Design review of the part shown in the three views and the two pictorial views. Dimensions are in mm from the part's minimum x, y and z. Round coordinates to 2 decimals unless told otherwise and drop trailing zeros. Write each loop counter-clockwise with the first axis right and the second up, starting at its lowest first coordinate (ties: lowest second). Pieces come first, ordered by that corner, then holes. Notation, with made-up numbers: (76, -4.75) -> (105, -4.75) arc R23 ccw to (105, 11.25) -> close; hole circle Ø11 at (52, 57). An arc over 180 degrees is marked (long way). Return JSON: item names as keys, results as strings. Group by question number.
1. Take a section at C-C, the plane x = 71.5. Write out the cut boundary in (y, z).
2. Take a section at B-B, the plane z = 27. Write out the cut boundary in (x, y).
3. Take a section at D-D, the plane y = 45.5. Write out the cut boundary in (x, z).
4. Take a section at A-A, the plane y = 27. Write out the cut boundary in (x, z).
5. Clearance check with flat-ended pins moving along their axes: P1, Ø5, axis at x = 98.5, z = 9.5, coming from the +Y side; P2, Ø3, axis at x = 69.5, y = 11, coming from the +Z side; P3, Ø4, axis at x = 71.5, y = 10, coming from the -Z side. State where each tip first meets the part, or that it passes through.
6. For line 1 along Z through (x, y) = (46, 27); line 2 along Y through (x, z) = (43, 17); line 3 along Z through (x, y) = (94.5, 33.5), list the stretches that pass through material, from the lowest coordinate up. Write a range as from..to.
7. Mouldability with a two-part tool opening along Y and no side actions: class the marked faces 1, 2 and 3 as pulls with the +Y half, pulls with the -Y half, needs draft (parallel to the pull), parting line crosses it, or undercut.
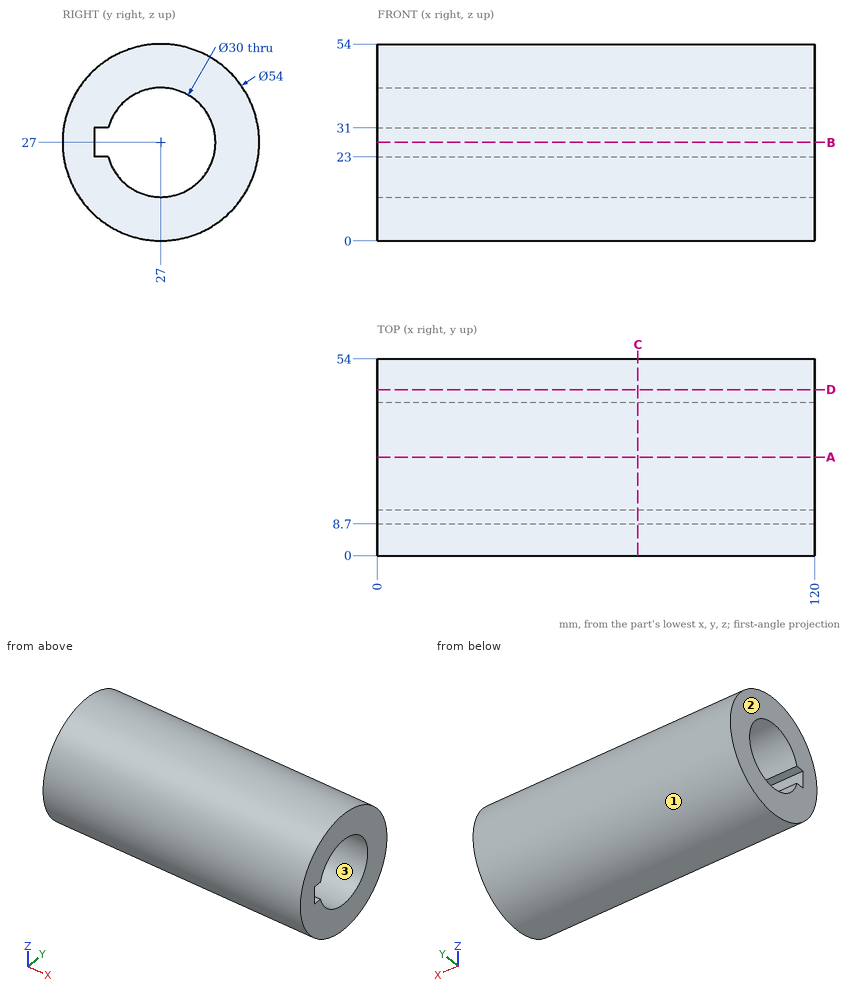
Output:
{
 "1": {"outline": "circle Ø54 at (27, 27); hole (8.7, 23) -> (12.54, 23) arc R15 ccw (long way) to (12.54, 31) -> (8.7, 31) -> close"},
 "2": {"outline": "(0, 0) -> (120, 0) -> (120, 8.7) -> (0, 8.7) -> close; (0, 42) -> (120, 42) -> (120, 54) -> (0, 54) -> close"},
 "3": {"outline": "(0, 7.33) -> (120, 7.33) -> (120, 46.67) -> (0, 46.67) -> close"},
 "4": {"outline": "(0, 0) -> (120, 0) -> (120, 12) -> (0, 12) -> close; (0, 42) -> (120, 42) -> (120, 54) -> (0, 54) -> close"},
 "5": {"P1": "stops at y = 49.45", "P2": "stops at z = 49.78", "P3": "stops at z = 4.55"},
 "6": {"line 1": "z = 0..12, 42..54", "line 2": "y = 1.92..15.82, 38.18..52.08", "line 3": "z = 0.79..13.48, 40.52..53.21"},
 "7": {"face 1": "parting line crosses it", "face 2": "needs draft", "face 3": "undercut"}
}
